from build123d import *

# Parameters (mm, degrees)
BOSS_EXTRUDE2_DEPTH = 0.5


with BuildPart() as part:
    # Sketch3 → Boss-Extrude2 (new body)
    with BuildSketch(Plane(origin=(0, 0, 0), x_dir=(1, 0, 0), z_dir=(0, 1, 0))):
        with BuildLine():
            ThreePointArc((-36.083785498, -43.43174801), (-46.924843817, -43.7399727), (-48.638393243, -54.449188186))
            add(Edge.make_bspline(
                [(-47.6612581, -69.620420628), (-44.67786304, -63.159473941), (-48.638393243, -54.449188186)],
                knots=[0, 0, 0, 1, 1, 1], degree=2))
            ThreePointArc((-47.6612581, -69.620420628), (-49.809928396, -74.901781564), (-48.13770816, -80.352766508))
            add(Edge.make_bspline(
                [(-48.794359492, -96.384204212), (-44.378776707, -88.222316074), (-48.13770816, -80.352766508)],
                knots=[0, 0, 0, 1, 1, 1], degree=2))
            ThreePointArc((-48.794359492, -96.384204212), (-43.404368002, -108.668799602), (-32.818291991, -100.428757923))
            add(Edge.make_bspline(
                [(-32.818291991, -100.428757923), (-30.846947347, -93.47063926), (-24.445798858, -94.793576843)],
                knots=[0, 0, 0, 1, 1, 1], degree=2))
            ThreePointArc((-24.445798858, -94.793576843), (-14.061121236, -94.354258183), (-11.865583386, -84.19482199))
            add(Edge.make_bspline(
                [(-13.164422653, -68.327872009), (-15.58680525, -74.860973905), (-11.865583386, -84.19482199)],
                knots=[0, 0, 0, 1, 1, 1], degree=2))
            ThreePointArc((-13.164422653, -68.327872009), (-11.067400095, -63.413067651), (-12.317814786, -58.217947961))
            add(Edge.make_bspline(
                [(-12.454215604, -42.252001936), (-17.252491187, -49.486356904), (-12.317814786, -58.217947961)],
                knots=[0, 0, 0, 1, 1, 1], degree=2))
            ThreePointArc((-12.454215604, -42.252001936), (-17.290607023, -29.356176902), (-28.026899399, -37.983170079))
            add(Edge.make_bspline(
                [(-36.083785498, -43.43174801), (-29.83167631, -44.511236738), (-28.026899399, -37.983170079)],
                knots=[0, 0, 0, 1, 1, 1], degree=2))
        make_face()
    extrude(amount=BOSS_EXTRUDE2_DEPTH)


solid = part.part
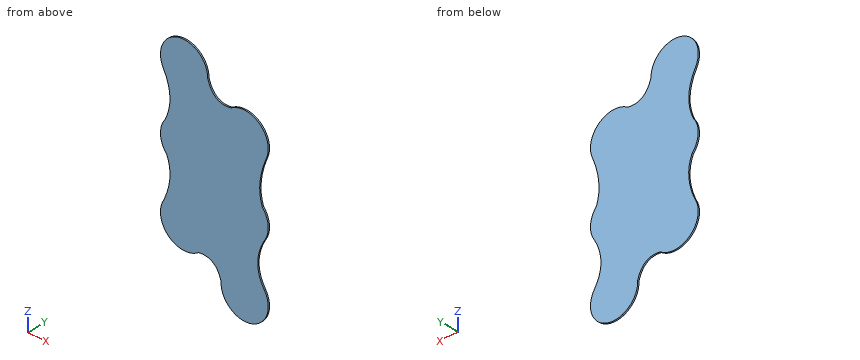
Source: CAD feature listing. Evaluate the final solid. Frame: model axes, mm. Give positions to 0.01 mm unless a question says otherwise; leave off trailing zeros. Loops run counter-clockwise (first coordinate to the right, second up) from the corner with the lowest first, then second, coordinate; pieces in that order, holes last. Notation, with made-up numbers: (59, -27.5) -> (118, -27.5) arc R21 cw to (118, -18.5) -> close; hole circle Ø7 at (81, 50.25). An arc over 180 degrees is marked (long way). Use a Markdown table: item, result. Add a question column.
1) Section query A-A, the plane x = -18. Return the cut outline in (y, z), then the cut area to 3 significant figures.
2) Line query: line 1 along Z through (x, y) = (-29, 0.45); line 2 along Z through (x, y) = (-34.5, 0.15); line 3 along X through (y, z) = (0.4, 91). Output: solid intervals per line, ascending. Write a range as [from, to].
3) Section query B-B, the plane x = -37. Return the cut outline in (y, z), then the cut area to 3 significant figures.
Numbers:
| question | item | result |
|---|---|---|
| 1 | outline | (0, 29.19) -> (0.5, 29.19) -> (0.5, 96.21) -> (0, 96.21) -> close |
| 1 | area | 33.5 mm2 |
| 2 | line 1 | z = [40.42, 95.12] |
| 2 | line 2 | z = [43.58, 105.5] |
| 2 | line 3 | x = [-46.76, -11.64] |
| 3 | outline | (0, 42.81) -> (0.5, 42.81) -> (0.5, 107.75) -> (0, 107.75) -> close |
| 3 | area | 32.5 mm2 |
